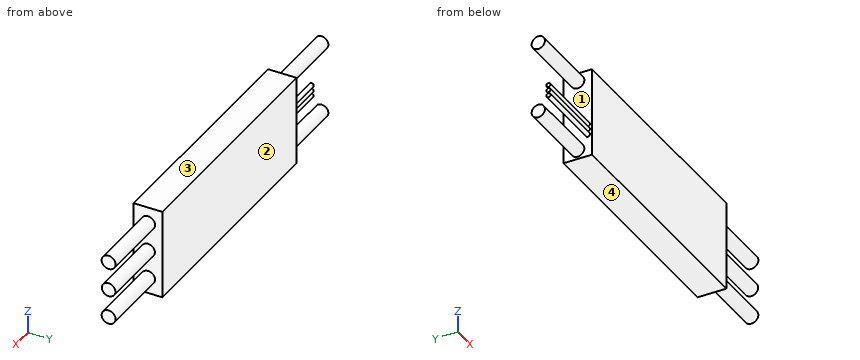
```python
from build123d import *

# Parameters (mm, degrees)
ESQUISSE1_W        = 68
ESQUISSE1_H        = 25
BOSS_EXTRU_1_DEPTH = 8
ESQUISSE2_R        = 1.85
ESQUISSE2_R_2      = 0.6
BOSS_EXTRU_2_DEPTH = 20
ESQUISSE3_R        = 1.945702626
ESQUISSE3_R_2      = 1.891437126
BOSS_EXTRU_3_DEPTH = 20


with BuildPart() as part:
    # Esquisse1 → Boss.-Extru.1 (new body)
    with BuildSketch(Plane(origin=(0, 0, 0), x_dir=(1, 0, 0), z_dir=(0, 1, 0))):
        Rectangle(ESQUISSE1_W, ESQUISSE1_H)
    extrude(amount=BOSS_EXTRU_1_DEPTH)

    # Esquisse2 → Boss.-Extru.2 (add)
    with BuildSketch(Plane.ZY.offset(34)):
        with Locations(Location((-10, 4, 0), (0, 0, 180))):
            Circle(ESQUISSE2_R)
        with Locations(Location((10, 4, 0), (0, 0, 180))):
            Circle(ESQUISSE2_R)
        with Locations(Location((-6.30252834, 1.162523301, 0), (0, 0, 180))):
            Circle(ESQUISSE2_R_2)
        with Locations(Location((-4.80252834, 1.162523301, 0), (0, 0, 180))):
            Circle(ESQUISSE2_R_2)
        with Locations(Location((-3.30252834, 1.162523301, 0), (0, 0, 180))):
            Circle(ESQUISSE2_R_2)
    extrude(amount=BOSS_EXTRU_2_DEPTH)

    # Esquisse3 → Boss.-Extru.3 (add)
    with BuildSketch(Plane(origin=(34, 0, 0), x_dir=(0, 0, -1), z_dir=(1, 0, 0))):
        with Locations(Location((-8, 4, 0), (0, 0, 180))):
            Circle(ESQUISSE3_R)
        with Locations(Location((0, 4, 0), (0, 0, 180))):
            Circle(ESQUISSE3_R_2)
        with Locations(Location((8, 4, 0), (0, 0, 180))):
            Circle(ESQUISSE3_R)
    extrude(amount=BOSS_EXTRU_3_DEPTH)


solid = part.part
```
Source: CAD feature listing. Evaluate the final solid. Frame: model axes, mm. Face numbers are marked on the shaded views. Coordinates: 2 decimals unless noted, no trailing zeros. Write each loop counter-clockwise with the first axis right and the second up, starting at its lowest first coordinate (ties: lowest second). Pieces come first, ordered by that corner, then holes. Notation, with made-up numbers: (-4, 11.25) - (7, 11.25) arc R16 ccw to (7, 26.25) - close; hole circle Ø2 at (-5, 15.25). An arc over 180 degrees is marked (long way). Answer as a JSON object with one key per item and string values.
Q1. Section query B-B, the plane z = 0. Output: boundary loops of the cut face in (x, y), plus the area to 3 significant figures.
Ans:
{"outline": "(-34, 0) - (34, 0) - (34, 2.11) - (54, 2.11) - (54, 5.89) - (34, 5.89) - (34, 8) - (-34, 8) - close", "area": "620 mm2"}
Q2. Draft query along Z for the marked faces 1, 2, 3 and 4. Return one class per face: released by +Z, released by -Z, zero draft, split by the parting line, or undercut.
Ans:
{"face 1": "undercut", "face 2": "zero draft", "face 3": "released by +Z", "face 4": "released by -Z"}
Q3. Section query D-D, the plane z = 4.5. Output: boundary loops of the cut face in (x, y).
Ans:
{"outline": "(-34, 0) - (34, 0) - (34, 8) - (-34, 8) - close"}
Q4. Section query C-C, the plane y = 4. Output: boundary loops of the cut face in (x, z), plus the area to 3 significant figures.
Ans:
{"outline": "(-54, -11.85) - (-34, -11.85) - (-34, -12.5) - (34, -12.5) - (34, -9.95) - (54, -9.95) - (54, -6.05) - (34, -6.05) - (34, -1.89) - (54, -1.89) - (54, 1.89) - (34, 1.89) - (34, 6.05) - (54, 6.05) - (54, 9.95) - (34, 9.95) - (34, 12.5) - (-34, 12.5) - (-34, 11.85) - (-54, 11.85) - (-54, 8.15) - (-34, 8.15) - (-34, -8.15) - (-54, -8.15) - close", "area": "2,080 mm2"}
Q5. Material intervals for line 1 (X direction, y = 6.5, z = -10.25); line 2 (Y direction, x = 39.5, z = 0); line 3 (X direction, y = 5, z = 11.5), sorted ascending. Write a range as [from, to].
Ans:
{"line 1": "x = [-34, 34]", "line 2": "y = [2.11, 5.89]", "line 3": "x = [-54, 34]"}
Q6. Section query A-A, the plane x = 37. Output: boundary loops of the cut face in (y, z).
Ans:
{"outline": "circle Ø3.89 at (4, -8); circle Ø3.89 at (4, 8); circle Ø3.78 at (4, 0)"}
Q7. First-contact query: pin 1 Ø4 at (y, z) = (7, -4.5) entering from +X; pin 2 Ø3 at (y, z) = (2, -0.5) entering from +X; pin 3 Ø1.5 at (y, z) = (2, 8) entering from -X. Flat tips, straight axial feed; report the tip coordinate or a pass-through.
Ans:
{"pin 1": "stops at x = 34", "pin 2": "stops at x = 54", "pin 3": "stops at x = -34"}
